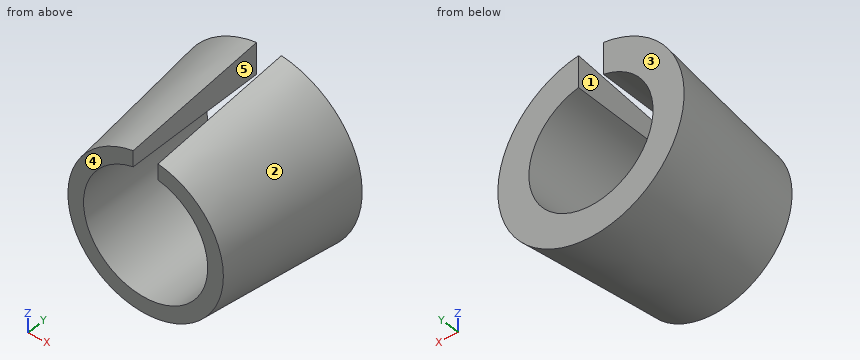
Autodesk Inventor part; units mm, degrees
ref_plane "YZ Plane" through (0, 0, 0) normal (1, 0, 0) x (0, 1, 0)
ref_plane "XZ Plane" through (0, 0, 0) normal (0, 1, 0) x (-1, 0, 0)
ref_plane "XY Plane" through (0, 0, 0) normal (0, 0, 1) x (1, 0, 0)
sketch "Skizze1" plane through (0, 0, 0) normal (0, 1, 0) x (-1, 0, 0)
  circle A0 centre (0, 0) radius 7.5
  dimension "d0" = 15
extrude "Extrusion1" add sketch "Skizze1" against normal blind 11.8
draft "Flächenverjüngung1" angle 6 pull direction (0, -1, 0) faces at (-7.4757, -7.8667, -0.6035) fixed edges at (7.5, 0, 0)
sketch "Skizze2" plane through (0, 0, 0) normal (0, 1, 0) x (1, 0, 0)
  circle A0 centre (0, 0) radius 7.5
hole "Bohrung1" at (0, 0, 0) direction (0, -1, 0) diameter 10 depth 11.8
sketch "Skizze4" plane through (0, 0, 0) normal (0, 1, 0) x (1, 0, 0)
  line L0 (1, -7.5) -> (-1, -7.5)
  line L1 (-1, -7.5) -> (-1, -4.899)
  line L2 (1, -4.899) -> (1, -7.5)
  circle A0 centre (0, 0) radius 5
  circle A1 centre (0, 0) radius 7.5
  point P0 (0, -7.5)
  point P1 (-1, -7.433)
  point P2 (1, -7.433)
  point P3 (0, -7.5)
  dimension "d12" = 2
extrude "Extrusion2" cut sketch "Skizze4" against normal up to surface (11.8 mm away) contours A1 L1 A0 L2 picked at (0, -5.8258)
properties part number "konus"
Build history of the part. All positions in model axes, mm. Face numbers are marked on the shaded views. A direction names the side the tool comes from. Give positions to 0.01 mm unless a question says otherwise; leave off trailing zeros. Order: outer loops, then holes, each group sorted by start corner. A loop starts at its lowest first (then second) coordinate and runs counter-clockwise, first axis right, second up. Notation, with made-up numbers: M 33,21 L 67,21 A19 ccw 67,40 Z; hole C 9.25,39.25 d10. An arc over 180 degrees is marked long. Use one line per item in the form item = value.
1) Saw through at B-B (x = 0). Give the cut face in (y, z).
Calculated:
outline = M -11.8,-6.26 L 0,-7.5 L 0,-5 L -11.8,-5 Z
2) Probe probe 1 along X at (y, z) = (-0.75, 0.5); probe 2 along X at (y, z) = (-9.5, -0.5); probe 3 along Z at (x, y) = (-1.5, -3.5). List the from-to ranges inside material, lowest first.
Calculated:
probe_1 = -7.4 to -4.97, 4.97 to 7.4
probe_2 = -6.48 to -4.97, 4.97 to 6.48
probe_3 = -6.97 to -4.77, 4.77 to 6.97
3) Tool access for the marked faces 4 and 5: list every direction of +Z, -Z, +X, -X, +Y, -Y with a clear straight run to the whole face (end or side of a thin tool).
Calculated:
face_4 = +Z, -Z, +X, -X, -Y
face_5 = +Z, +Y, -Y
4) Drop flat-ended pins along their axis: pin 1 (5 mm diameter, centred on x = -2, y = -8, fed in from -Z); pin 2 (1.3 mm diameter, centred on y = -6.5, z = 6, fed in from -X); pin 3 (8 mm diameter, centred on x = 0, z = 0, fed in from -Y); pin 4 (3 mm diameter, centred on y = -5.5, z = 3.5, fed in from +X). Give the stop position or say it passes through.
Calculated:
pin_1 = -6.85
pin_2 = -4.23
pin_3 = through
pin_4 = 6.66
5) Two-plate mould, pull along X, no slides. Class the marked faces 1, 2 and 3: released by +X, released by -X, zero draft, split by the parting line, or undercut.
Calculated:
face_1 = undercut
face_2 = split by the parting line
face_3 = zero draft
6) Saw through at A-A (z = 0). Give the cut face in (x, y).
Calculated:
outline = M -7.5,0 L -6.26,-11.8 L -5,-11.8 L -5,0 Z; M 5,-11.8 L 6.26,-11.8 L 7.5,0 L 5,0 Z
7) Saw through at C-C (y = -7.5). Give the cut face in (x, z), plus the area to 3 significant figures.
Calculated:
outline = M -1,4.9 L -1,6.64 A6.71 ccw long 1,6.64 L 1,4.9 A5 cw long Z
area = 59.5 mm2
